from build123d import *

# Parameters (mm, degrees)
ESQUISSE1_R             = 3.5
ESQUISSE1_R_2           = 1.5
BOSS_EXTRU_1_DEPTH      = 2
ESQUISSE2_R             = 2.5
ESQUISSE2_R_2           = 1.5
BOSS_EXTRU_2_DEPTH      = 3
ESQUISSE3_R             = 1.5
BOSS_EXTRU_3_DEPTH      = 8.5
ESQUISSE4_R             = 2.5
BOSS_EXTRU_4_DEPTH      = 8
ESQUISSE5_R             = 2.5
ENL_V_MAT_EXTRU_1_DEPTH = 12


with BuildPart() as part:
    # Esquisse1 → Boss.-Extru.1 (new body)
    with BuildSketch(Plane(origin=(0, 0, 0), x_dir=(1, 0, 0), z_dir=(0, 1, 0))):
        Circle(ESQUISSE1_R)
        Circle(ESQUISSE1_R_2, mode=Mode.SUBTRACT)
    extrude(amount=BOSS_EXTRU_1_DEPTH)

    # Esquisse2 → Boss.-Extru.2 (add)
    with BuildSketch(Plane(origin=(0, 2, 0), x_dir=(1, 0, 0), z_dir=(0, 1, 0))):
        Circle(ESQUISSE2_R)
        Circle(ESQUISSE2_R_2, mode=Mode.SUBTRACT)
    extrude(amount=BOSS_EXTRU_2_DEPTH)

    # Esquisse3 → Boss.-Extru.3 (add)
    with BuildSketch(Plane(origin=(0, 5, 0), x_dir=(1, 0, 0), z_dir=(0, 1, 0))):
        Polygon((-6, 3.464101615), (-6, -3.464101615), (0, -6.92820323), (6, -3.464101615), (6, 3.464101615), (0, 6.92820323), align=None)
        Circle(ESQUISSE3_R, mode=Mode.SUBTRACT)
    extrude(amount=BOSS_EXTRU_3_DEPTH)

    # Esquisse4 → Boss.-Extru.4 (add)
    with BuildSketch(Plane(origin=(0, 13.5, 0), x_dir=(1, 0, 0), z_dir=(0, 1, 0))):
        Circle(ESQUISSE4_R)
    extrude(amount=BOSS_EXTRU_4_DEPTH)

    # Esquisse5 → Enlèv. mat.-Extru.1 (cut)
    with BuildSketch(Plane.ZY.offset(6)):
        with Locations((0, 9.25)):
            Circle(ESQUISSE5_R)
    extrude(amount=-ENL_V_MAT_EXTRU_1_DEPTH, mode=Mode.SUBTRACT)


solid = part.part
Model file for the job. Use its own axes, mm. A direction names the side the tool comes from. Give positions to 0.01 mm unless a question says otherwise; leave off trailing zeros. Order: outer loops, then holes, each group sorted by start corner. A loop starts at its lowest first (then second) coordinate and runs counter-clockwise, first axis right, second up. Notation, with made-up numbers: (42, 80.5) - (49, 80.5) arc R25 ccw to (49, 109.5) - close; hole circle Ø3 at (13, 54). An arc over 180 degrees is marked (long way). One line per item, written item: value.
Item 1: Tool access for faces 1 (the flat face through (2, 2, 2)), 2 (the cylindrical face through (-0.325, 3.574, 1.464)), 3 (the cylindrical face through (-0.54, 17.44, 2.44)): list every direction of +Z, -Z, +X, -X, +Y, -Y with a clear straight run to the whole face (end or side of a thin tool).
Response values:
face 1: none
face 2: -Y
face 3: +Y
Item 2: Slice it at C-C (y = 9.25). List the corners of the cut face in (x, z).
Response values:
outline: (-6, -3.46) - (0, -6.93) - (6, -3.46) - (6, -2.5) - (-6, -2.5) - close; (-6, 2.5) - (6, 2.5) - (6, 3.46) - (0, 6.93) - (-6, 3.46) - close
Item 3: Two-plate mould, pull along Y, no slides. Class faces 4 (the flat face through (0, 13.5, 0)), 5 (the flat face through (0, 13.5, 3)), 6 (the flat face through (-2.96, 9.19, -5.22)), 7 (the cylindrical face through (-0.54, 3.48, 2.44)): released by +Y, released by -Y, zero draft, split by the parting line, or undercut.
Response values:
face 4: released by -Y
face 5: released by +Y
face 6: zero draft
face 7: undercut
Item 4: Slice it at D-D (z = 0). List the corners of the cut face in (x, y).
Response values:
outline: (-6, 5) - (-2.5, 5) - (-2.5, 2) - (-3.5, 2) - (-3.5, 0) - (-1.5, 0) - (-1.5, 6.75) - (-6, 6.75) - close; (-6, 11.75) - (-1.5, 11.75) - (-1.5, 13.5) - (1.5, 13.5) - (1.5, 11.75) - (6, 11.75) - (6, 13.5) - (2.5, 13.5) - (2.5, 21.5) - (-2.5, 21.5) - (-2.5, 13.5) - (-6, 13.5) - close; (1.5, 0) - (3.5, 0) - (3.5, 2) - (2.5, 2) - (2.5, 5) - (6, 5) - (6, 6.75) - (1.5, 6.75) - close
Item 5: Slice it at A-A (y = 12.75). List the corners of the cut face in (x, z).
Response values:
outline: (-6, -3.46) - (0, -6.93) - (6, -3.46) - (6, 3.46) - (0, 6.93) - (-6, 3.46) - close; hole circle Ø3 at (0, 0)
Item 6: Pin check, flat tips, straight feed: pin 1 Ø1.5 at (x, z) = (4, 4) entering from -Y; pin 2 Ø2.5 at (x, z) = (0, 0) entering from -Y; pin 3 Ø3 at (y, z) = (2.5, -1) entering from +X. Stop position of each tip, or through.
Response values:
pin 1: y = 5
pin 2: y = 13.5
pin 3: x = 3.5
Item 7: Slice it at B-B (x = -2.75). List the corners of the cut face in (y, z), then the cut area to 3 significant figures.
Response values:
outline: (0, -2.17) - (2, -2.17) - (2, 2.17) - (0, 2.17) - close; (5, -5.34) - (13.5, -5.34) - (13.5, 5.34) - (5, 5.34) - close; hole circle Ø5 at (9.25, 0)
area: 79.8 mm2
Item 8: Wall check: line 1 (Y direction, x = -2.75, z = 0); line 2 (X direction, y = 2.5, z = 0); line 3 (X direction, y = 20.75, z = 0). Give the ranges that are in metal, low to high.
Response values:
line 1: 0 to 2, 5 to 6.75, 11.75 to 13.5
line 2: -2.5 to -1.5, 1.5 to 2.5
line 3: -2.5 to 2.5
